Check sheet for the modelled part. Datum: model origin and axes. Units: mm. Give positions to 0.01 mm unless a question says otherwise; leave off trailing zeros. Order: outer loops, then holes, each group sorted by start corner. A loop starts at its lowest first (then second) coordinate and runs counter-clockwise, first axis right, second up.
```python
from build123d import *

# Parameters (mm, degrees)
CROQUIS1_W              = 200
CROQUIS1_H              = 190
SALIENTE_EXTRUIR1_DEPTH = 3
CORTAR_EXTRUIR1_DEPTH   = 3


with BuildPart() as part:
    # Croquis1 → Saliente-Extruir1 (new body)
    with BuildSketch(Plane.XY):
        Rectangle(CROQUIS1_W, CROQUIS1_H)
    extrude(amount=SALIENTE_EXTRUIR1_DEPTH)

    # Croquis2 → Cortar-Extruir1 (cut)
    with BuildSketch(Plane.XY.offset(3)):
        with BuildLine():
            Line((5, 12.5), (-100, 12.5))
            Line((-100, 12.5), (-100, 0))
            Line((-100, 0), (-100, -12.5))
            Line((-100, -12.5), (5, -12.5))
            ThreePointArc((5, -12.5), (17.5, 0), (5, 12.5))
        make_face()
    extrude(amount=-CORTAR_EXTRUIR1_DEPTH, mode=Mode.SUBTRACT)


solid = part.part
```
(1) Cross-section at B-B on z = 1.55. Enter the section's corners in (x, y).
Response values:
outline: (-100, -95) - (100, -95) - (100, 95) - (-100, 95) - (-100, 12.5) - (5, 12.5) arc R12.5 cw to (5, -12.5) - (-100, -12.5) - close
(2) Cross-section at C-C on y = 0. Enter the section's corners in (x, z), then the cut area to 4 significant figures.
Response values:
outline: (17.5, 0) - (100, 0) - (100, 3) - (17.5, 3) - close
area: 247.5 mm2
(3) Gauge pin test, flat end, axial feed: pin 1 Ø8 at (x, y) = (48, 53) entering from -Z. Record the tip position at first contact, or that the pin passes through.
Response values:
pin 1: stops at z = 0
(4) Cross-section at A-A on x = 2.5. Enter the section's corners in (y, z), then the cut area to 3 significant figures.
Response values:
outline: (-95, 0) - (-12.5, 0) - (-12.5, 3) - (-95, 3) - close; (12.5, 0) - (95, 0) - (95, 3) - (12.5, 3) - close
area: 495 mm2
(5) Material ranges on L1, parallel to Y at x = -63, z = 1.95; L2, parallel to X at y = 10, z = 0.4; L3, parallel to X at y = -0.5, z = 1.7, recorded low to high.
Response values:
L1: y = -95 to -12.5, 12.5 to 95
L2: x = 12.5 to 100
L3: x = 17.49 to 100
